from build123d import *
from OCP.BRepFilletAPI import BRepFilletAPI_MakeChamfer

# Parameters (mm, degrees)
SKETCH2_W           = 35.5
SKETCH2_H           = 35.6
BOSS_EXTRUDE1_DEPTH = 50.6
SKETCH3_R           = 11
BOSS_EXTRUDE2_DEPTH = 2.75
SKETCH4_R           = 3.9
BOSS_EXTRUDE3_DEPTH = 5.35
CHAMFER1_SIZE       = 6
CHAMFER1_SIZE2      = 5.1
MIRROR3_START       = -17.75
MIRROR3_DEPTH       = 35.5


# Read off the part's stored shape, not the designer's step: Mirror3
with BuildPart() as part:
    # Sketch2 → Boss-Extrude1 (new body)
    with BuildSketch(Plane(origin=(0, -12, 0), x_dir=(-1, 0, 0), z_dir=(0, 1, 0))):
        Rectangle(SKETCH2_W, SKETCH2_H)
    extrude(amount=BOSS_EXTRUDE1_DEPTH)

    # Sketch3 → Boss-Extrude2 (add)
    with BuildSketch(Plane(origin=(17.75, 0, 0), x_dir=(0, 0, -1), z_dir=(1, 0, 0))):
        with Locations(Location((0, 0, 0), (0, 0, 180))):
            Circle(SKETCH3_R)
    boss_extrude2 = extrude(amount=BOSS_EXTRUDE2_DEPTH)

    # Sketch4 → Boss-Extrude3 (add)
    with BuildSketch(Plane(origin=(20.5, 0, 0), x_dir=(0, 0, -1), z_dir=(1, 0, 0))):
        Circle(SKETCH4_R)
    boss_extrude3 = extrude(amount=BOSS_EXTRUDE3_DEPTH)

    # Chamfer1: one chamfer whose edges measure the first distance from different faces: ONE call of the kernel's chamfer builder (chamfer() names one face for all edges)
    chamfer1_edges_1 = [part.edges().sort_by_distance(p)[0] for p in [
        (0, 38.6, -17.8),
    ]]
    chamfer1_side_1 = [part.faces().sort_by_distance(p)[0] for p in [
        (0, 13.3, -17.8),
    ]]
    chamfer1_edges_2 = [part.edges().sort_by_distance(p)[0] for p in [
        (0, 38.6, 17.8),
    ]]
    chamfer1_side_2 = [part.faces().sort_by_distance(p)[0] for p in [
        (0, 13.3, 17.8),
    ]]
    chamfer1 = BRepFilletAPI_MakeChamfer(part.part.solid().wrapped)
    for e in chamfer1_edges_1:
        chamfer1.Add(CHAMFER1_SIZE, CHAMFER1_SIZE2, e.wrapped, chamfer1_side_1[0].wrapped)  # the first distance lies on this face
    for e in chamfer1_edges_2:
        chamfer1.Add(CHAMFER1_SIZE, CHAMFER1_SIZE2, e.wrapped, chamfer1_side_2[0].wrapped)  # the first distance lies on this face
    add(Compound.cast(chamfer1.Shape()), mode=Mode.REPLACE)

    # Mirror1: Boss-Extrude2, Boss-Extrude3 across plane
    add(boss_extrude2.mirror(Plane(origin=(0, 0, 0), x_dir=(0, 0, 1), z_dir=(1, 0, 0))))
    add(boss_extrude3.mirror(Plane(origin=(0, 0, 0), x_dir=(0, 0, 1), z_dir=(1, 0, 0))))

    # Mirror3 outline → Mirror3 (cut)
    with BuildSketch(Plane.YZ.offset(MIRROR3_START)):
        Polygon((-6, -17.8), (-12, -12.7), (-12, -17.8), align=None)
        Polygon((-12, 12.7), (-6, 17.8), (-12, 17.8), align=None)
    extrude(amount=MIRROR3_DEPTH, mode=Mode.SUBTRACT)


solid = part.part
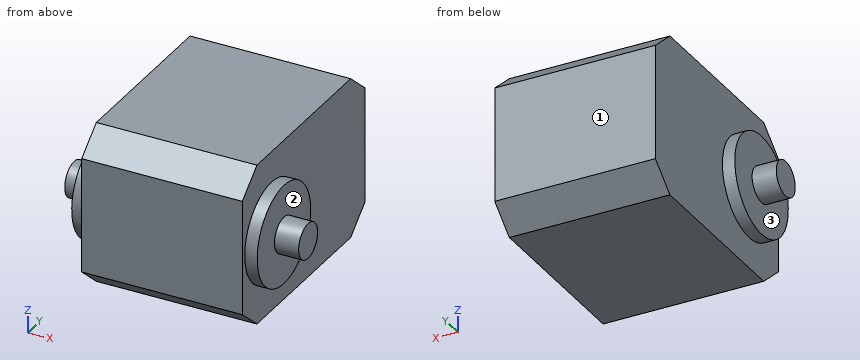
Input: part model. Units: mm. Frame: model coordinates. Face numbers are marked on the shaded views. A direction names the side the tool comes from. Give positions to 0.01 mm unless a question says otherwise; leave off trailing zeros. Order: outer loops, then holes, each group sorted by start corner. A loop starts at its lowest first (then second) coordinate and runs counter-clockwise, first axis right, second up. Notation, with made-up numbers: (13.5, 70.25) - (64.5, 70.25) arc R31 ccw to (64.5, 105.25) - close; hole circle Ø3 at (-32.5, 39.25). An arc over 180 degrees is marked (long way). Answer as a JSON object with one key per item and string values. Group by question number.
Q1. Cut plane A-A, the plane y = 0. Output: boundary loops of the cut face in (x, z), then the cut area to 3 significant figures.
Q2. Cut plane B-B, the plane z = 0. Output: boundary loops of the cut face in (x, y).
Q3. Cut plane D-D, the plane x = 21.5. Output: boundary loops of the cut face in (y, z).
Q4. Set-up query: the marked faces 1, 2 and 3. Return all of +Z, -Z, +X, -X, +Y, -Y with unobstructed straight access to the full face (end or side cutting, diameter ignored); none if empty.
Q5. First-contact query: pin 1 Ø6 at (y, z) = (11, 12) entering from -X; pin 2 Ø1.5 at (y, z) = (30.5, -5) entering from +X. Flat tips, straight axial feed; report the tip coordinate or a pass-through.
Q6. Line query: probe 1 along X at (y, z) = (4, -3.5); probe 2 along X at (y, z) = (2.5, -11); probe 3 along Z at (x, y) = (-14.5, -10). Output: solid intervals per line, ascending.
Q7. Cut plane C-C, the plane x = 0. Output: boundary loops of the cut face in (y, z).
Results:
{
 "1": {"outline": "(-25.85, -3.9) - (-20.5, -3.9) - (-20.5, -11) - (-17.75, -11) - (-17.75, -17.8) - (17.75, -17.8) - (17.75, -11) - (20.5, -11) - (20.5, -3.9) - (25.85, -3.9) - (25.85, 3.9) - (20.5, 3.9) - (20.5, 11) - (17.75, 11) - (17.75, 17.8) - (-17.75, 17.8) - (-17.75, 11) - (-20.5, 11) - (-20.5, 3.9) - (-25.85, 3.9) - close", "area": "1,470 mm^2"},
 "2": {"outline": "(-25.85, -3.9) - (-20.5, -3.9) - (-20.5, -11) - (-17.75, -11) - (-17.75, -12) - (17.75, -12) - (17.75, -11) - (20.5, -11) - (20.5, -3.9) - (25.85, -3.9) - (25.85, 3.9) - (20.5, 3.9) - (20.5, 11) - (17.75, 11) - (17.75, 38.6) - (-17.75, 38.6) - (-17.75, 11) - (-20.5, 11) - (-20.5, 3.9) - (-25.85, 3.9) - close"},
 "3": {"outline": "circle Ø7.8 at (0, 0)"},
 "4": {"face 1": "+Z, -Z, +X, -X, +Y", "face 2": "+X", "face 3": "-X"},
 "5": {"pin 1": "x = -17.75", "pin 2": "x = 17.75"},
 "6": {"probe 1": "-20.5 to 20.5", "probe 2": "-17.75 to 17.75", "probe 3": "-14.4 to 14.4"},
 "7": {"outline": "(-12, -12.7) - (-6, -17.8) - (32.6, -17.8) - (38.6, -12.7) - (38.6, 12.7) - (32.6, 17.8) - (-6, 17.8) - (-12, 12.7) - close"}
}
